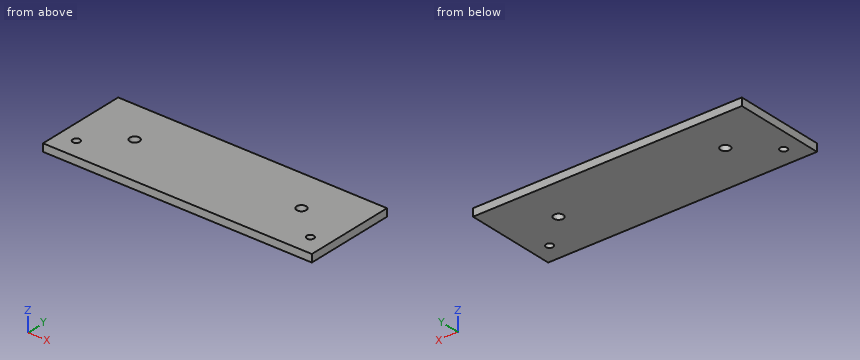
```python
from build123d import *

# Parameters (mm, degrees)
SKETCH1_W           = 224
SKETCH1_H           = 76.2
SKETCH1_R           = 4
SKETCH1_R_2         = 3
BOSS_EXTRUDE1_DEPTH = 6.35


with BuildPart() as part:
    # Sketch1 → Boss-Extrude1 (new body)
    with BuildSketch(Plane.XY):
        with Locations((112, 38.1)):
            Rectangle(SKETCH1_W, SKETCH1_H)
        with Locations((42.5, 41.2)):
            Circle(SKETCH1_R, mode=Mode.SUBTRACT)
        with Locations((181.5, 41.2)):
            Circle(SKETCH1_R, mode=Mode.SUBTRACT)
        with Locations((14.5, 16.2)):
            Circle(SKETCH1_R_2, mode=Mode.SUBTRACT)
        with Locations((209.5, 16.2)):
            Circle(SKETCH1_R_2, mode=Mode.SUBTRACT)
    extrude(amount=BOSS_EXTRUDE1_DEPTH)


solid = part.part
```
Could you check a few things on this model? Use its own coordinates, in mm. Give positions to 0.01 mm unless a question says otherwise; leave off trailing zeros. Write each loop counter-clockwise with the first axis right and the second up, starting at its lowest first coordinate (ties: lowest second). Pieces come first, ordered by that corner, then holes. Notation, with made-up numbers: (62.25, 41) -> (79.25, 41) arc R23 ccw to (79.25, 49) -> close; hole circle Ø11 at (76.25, -4). An arc over 180 degrees is marked (long way). Write each question's results on one line, items separated by ' | '.
1. I want a section at B-B, the plane y = 41.2. Write out the boundary of the cut face in (x, z).
Check sheet entries:
outline: (0, 0) -> (38.5, 0) -> (38.5, 6.35) -> (0, 6.35) -> close; (46.5, 0) -> (177.5, 0) -> (177.5, 6.35) -> (46.5, 6.35) -> close; (185.5, 0) -> (224, 0) -> (224, 6.35) -> (185.5, 6.35) -> close
2. I want a section at A-A, the plane x = 181.5. Write out the boundary of the cut face in (y, z).
Check sheet entries:
outline: (0, 0) -> (37.2, 0) -> (37.2, 6.35) -> (0, 6.35) -> close; (45.2, 0) -> (76.2, 0) -> (76.2, 6.35) -> (45.2, 6.35) -> close
3. I need wall thicknesses on L1, parallel to Y at x = 209, z = 0.5; L2, parallel to Y at x = 42.5, z = 3.25; L3, parallel to X at y = 15.5, z = 4. Which ranges of each line are inside material? Lowest first, please.
Check sheet entries:
L1: y = 0 to 13.24, 19.16 to 76.2 | L2: y = 0 to 37.2, 45.2 to 76.2 | L3: x = 0 to 11.58, 17.42 to 206.58, 212.42 to 224
